```python
from build123d import *

# Parameters (mm, degrees)
BASE_FLANGE1_DEPTH = 490.75


# Sheet-metal steps are written as plain solids
with BuildPart() as part:
    # Sketch1 → Base-Flange1 (new, symmetric)
    with BuildSketch(Plane(origin=(0, 0, 0), x_dir=(1, 0, 0), z_dir=(0, 1, 0))):
        with BuildLine():
            Line((9.5, 59.25), (9.5, 68.0134))
            ThreePointArc((9.5, 68.0134), (10.081861668, 69.418138332), (11.4866, 70))
            Line((11.4866, 70), (37.5134, 70))
            ThreePointArc((37.5134, 70), (38.918138332, 69.418138332), (39.5, 68.0134))
            Line((39.5, 68.0134), (39.5, 23))
            Line((39.5, 23), (39.5, 8.562771629))
            ThreePointArc((39.5, 8.562771629), (39.724914644, 8.032905932), (40.262306969, 7.826620346))
            Line((40.262306969, 7.826620346), (42.153527557, 7.892663224))
            ThreePointArc((42.153527557, 7.892663224), (42.675221066, 8.135932903), (42.862626267, 8.680197126))
            Line((42.862626267, 8.680197126), (42.359529101, 15.874821789))
            ThreePointArc((42.359529101, 15.874821789), (42.88838258, 17.368257942), (44.341289843, 18))
            Line((44.341289843, 18), (52.2634, 18))
            ThreePointArc((52.2634, 18), (53.668138332, 17.418138332), (54.25, 16.0134))
            Line((54.25, 16.0134), (54.25, -23))
            Line((54.25, -23), (54.25, -68.0134))
            ThreePointArc((54.25, -68.0134), (53.668138332, -69.418138332), (52.2634, -70))
            Line((52.2634, -70), (39.5, -70))
            Line((39.5, -70), (11.4866, -70))
            ThreePointArc((11.4866, -70), (10.081861668, -69.418138332), (9.5, -68.0134))
            Line((9.5, -68.0134), (9.5, -59.25))
            Line((9.5, -59.25), (10.75, -59.25))
            Line((10.75, -59.25), (10.75, -68.0134))
            ThreePointArc((10.75, -68.0134), (10.965745145, -68.534254855), (11.4866, -68.75))
            Line((11.4866, -68.75), (39.5, -68.75))
            Line((39.5, -68.75), (52.2634, -68.75))
            ThreePointArc((52.2634, -68.75), (52.784254855, -68.534254855), (53, -68.0134))
            Line((53, -68.0134), (53, -23))
            Line((53, -23), (53, 16.0134))
            ThreePointArc((53, 16.0134), (52.784254855, 16.534254855), (52.2634, 16.75))
            Line((52.2634, 16.75), (44.341289843, 16.75))
            ThreePointArc((44.341289843, 16.75), (43.802574707, 16.515759992), (43.606484164, 15.962017381))
            Line((43.606484164, 15.962017381), (44.10958133, 8.767392718))
            ThreePointArc((44.10958133, 8.767392718), (43.604152098, 7.299519645), (42.197151928, 6.64342469))
            Line((42.197151928, 6.64342469), (40.30593134, 6.577381812))
            ThreePointArc((40.30593134, 6.577381812), (38.856591681, 7.133731182), (38.25, 8.562771629))
            Line((38.25, 8.562771629), (38.25, 23))
            Line((38.25, 23), (38.25, 68.0134))
            ThreePointArc((38.25, 68.0134), (38.034254855, 68.534254855), (37.5134, 68.75))
            Line((37.5134, 68.75), (11.4866, 68.75))
            ThreePointArc((11.4866, 68.75), (10.965745145, 68.534254855), (10.75, 68.0134))
            Line((10.75, 68.0134), (10.75, 59.25))
            Line((10.75, 59.25), (9.5, 59.25))
        make_face()
    extrude(amount=BASE_FLANGE1_DEPTH, both=True)


solid = part.part
```
Source: CAD feature listing. Evaluate the final solid. Frame: model axes, mm. A direction names the side the tool comes from. Coordinates: 2 decimals unless noted, no trailing zeros. Write each loop counter-clockwise with the first axis right and the second up, starting at its lowest first coordinate (ties: lowest second). Pieces come first, ordered by that corner, then holes. Notation, with made-up numbers: M 0,62 L 59,62 A22 ccw 59,88 Z; hole C -6.75,63.25 d6. An arc over 180 degrees is marked long. Answer as a JSON object with one key per item and string values.
1. Contact query for flat-ended pins moving along their axis: P1, Ø18, axis at y = -101.5, z = -41.5, coming from the -X side; P2, Ø6.5, axis at x = 50, y = -188, coming from the -Z side; P3, Ø2, axis at y = -391, z = 25.5, coming from the -X side. Output: stop coordinate, or through.
Evaluation:
{"P1": "x = 38.25", "P2": "z = -18", "P3": "x = 53"}
2. Cut plane A-A on x = 20.5. Output: boundary loops of the cut face in (y, z), plus the area to 3 significant figures.
Evaluation:
{"outline": "M -490.75,-70 L 490.75,-70 L 490.75,-68.75 L -490.75,-68.75 Z; M -490.75,68.75 L 490.75,68.75 L 490.75,70 L -490.75,70 Z", "area": "2,450 mm^2"}
3. Draft query along Z for faces 1 (the flat face through (54.25, 7, 25)), 2 (the flat face through (38.25, 7, -38)), 3 (the flat face through (32, 7, 70)). Return one class per face: released by +Z, released by -Z, zero draft, split by the parting line, or undercut.
Evaluation:
{"face 1": "zero draft", "face 2": "undercut", "face 3": "released by +Z"}
4. Access query for faces 4 (the flat face through (43.6, -490.75, -10.7)), 5 (the flat face through (53, 7, 27)). Directions: +Z, -Z, +X, -X, +Y, -Y. A direction counts if a zero-diameter tool reaches every point of the face in a straight line with its end or side. Return the directions, or none.
Evaluation:
{"face 4": "+Z, -Z, +X, -X, -Y", "face 5": "+Y, -Y"}
5. Cut plane B-B on z = 30. Output: boundary loops of the cut face in (x, y), plus the area to 3 significant figures.
Evaluation:
{"outline": "M 53,-490.75 L 54.25,-490.75 L 54.25,490.75 L 53,490.75 Z", "area": "1,230 mm^2"}
6. Ray query, L1, parallel to Z at x = 30, y = -248; L2, parallel to Z at x = 41, y = 420; L3, parallel to X at y = -373.5, z = -60.5. Return the intervals inside material, ascending.
Evaluation:
{"L1": "-70 to -68.75, 68.75 to 70", "L2": "-7.85 to -6.6, 68.75 to 70", "L3": "9.5 to 10.75, 38.25 to 39.5"}
